Check sheet for the modelled part. Datum: model origin and axes. Units: mm. A direction names the side the tool comes from. Give positions to 0.01 mm unless a question says otherwise; leave off trailing zeros. Loops run counter-clockwise (first coordinate to the right, second up) from the corner with the lowest first, then second, coordinate; pieces in that order, holes last. Notation, with made-up numbers: (0.5, 2.25) - (4.5, 2.25) arc R23 ccw to (4.5, 17.25) - close; hole circle Ø4 at (-38, 84.25). An arc over 180 degrees is marked (long way). Use CSV: the item, a comma, the result in double quotes.
from build123d import *

# Parameters (mm, degrees)
SKETCH_R  = 1.7
PAD_DEPTH = 3


with BuildPart() as part:
    # Sketch → Pad (new body)
    with BuildSketch(Plane.XY):
        with BuildLine():
            ThreePointArc((-11.338775, -5.261385), (-11.137582, -5.674881), (-10.921315, -6.080698))
            Line((-10.921315, -6.080698), (-12.869031, -8.11383))
            ThreePointArc((-12.869031, -8.11383), (-12.957339, -9.414058), (-11.69346, -9.731864))
            Line((-11.69346, -9.731864), (-9.157959, -8.507749))
            ThreePointArc((-9.157959, -8.507749), (-8.838835, -8.838835), (-8.507749, -9.157959))
            Line((-8.507749, -9.157959), (-9.731864, -11.69346))
            ThreePointArc((-9.731864, -11.69346), (-9.414058, -12.957339), (-8.11383, -12.869031))
            Line((-8.11383, -12.869031), (-6.080698, -10.921315))
            ThreePointArc((-6.080698, -10.921315), (-5.674881, -11.137582), (-5.261385, -11.338775))
            Line((-5.261385, -11.338775), (-5.642075, -14.128453))
            ThreePointArc((-5.642075, -14.128453), (-4.949263, -15.232265), (-3.739962, -14.746487))
            Line((-3.739962, -14.746487), (-2.408215, -12.265826))
            ThreePointArc((-2.408215, -12.265826), (-1.955431, -12.346104), (-1.5, -12.409674))
            Line((-1.5, -12.409674), (-1, -15.180455))
            ThreePointArc((-1, -15.180455), (0, -16.016151), (1, -15.180455))
            Line((1, -15.180455), (1.5, -12.409674))
            ThreePointArc((1.5, -12.409674), (7.008593, -10.350344), (10.965856, -6))
            Line((30.259157, -5), (10.965856, -6))
            ThreePointArc((30.259157, -5), (35.006712, 0), (30.259157, 5))
            Line((10.965856, 6), (30.259157, 5))
            ThreePointArc((10.965856, 6), (-0.413709, 12.493152), (-11.338775, 5.261385))
            Line((-11.338775, 5.261385), (-14.128453, 5.642075))
            ThreePointArc((-14.128453, 5.642075), (-15.232265, 4.949263), (-14.746487, 3.739962))
            Line((-14.746487, 3.739962), (-12.265826, 2.408215))
            ThreePointArc((-12.265826, 2.408215), (-12.346104, 1.955431), (-12.409674, 1.5))
            Line((-12.409674, 1.5), (-15.180455, 1))
            ThreePointArc((-15.180455, 1), (-16.016151, 0), (-15.180455, -1))
            Line((-15.180455, -1), (-12.409674, -1.5))
            ThreePointArc((-12.409674, -1.5), (-12.346104, -1.955431), (-12.265826, -2.408215))
            Line((-12.265826, -2.408215), (-14.746487, -3.739962))
            ThreePointArc((-14.746487, -3.739962), (-15.232265, -4.949263), (-14.128453, -5.642075))
            Line((-14.128453, -5.642075), (-11.338775, -5.261385))
        make_face()
        Circle(SKETCH_R, mode=Mode.SUBTRACT)
        with Locations((7, 0)):
            Circle(SKETCH_R, mode=Mode.SUBTRACT)
        with Locations((-7, 0)):
            Circle(SKETCH_R, mode=Mode.SUBTRACT)
        with Locations((30, 0)):
            Circle(SKETCH_R, mode=Mode.SUBTRACT)
    extrude(amount=PAD_DEPTH)


solid = part.part
1. Release check for a two-part mould opening along Y. For faces 4 (the face through (-8.35, -1.03, 1.48)), 5 (the face through (-0.2, 12.5, 1.5)), 6 (the face through (-1.962, -12.345, 1.479)) record: released by +Y, released by -Y, zero draft, split by the parting line, or undercut.
Completed:
face 4,"undercut"
face 5,"released by +Y"
face 6,"released by -Y"
2. Sectioned sample at C-C, the plane z = 0.6. State how many separate pieces and enclosed holes the cut face has, and give its area (3 significant figures).
Completed:
separate pieces,"1"
enclosed holes,"4"
area,"747 mm²"
3. Sectioned sample at A-A, the plane x = 0. Record the boundary of the cut face in (y, z).
Completed:
outline,"(-16.02, 0) - (-1.7, 0) - (-1.7, 3) - (-16.02, 3) - close; (1.7, 0) - (12.5, 0) - (12.5, 3) - (1.7, 3) - close"
4. Sectioned sample at D-D, the plane x = -7.5. Record the boundary of the cut face in (y, z).
Completed:
outline,"(-12.28, 0) - (-1.62, 0) - (-1.62, 3) - (-12.28, 3) - close; (1.62, 0) - (10, 0) - (10, 3) - (1.62, 3) - close"
5. Set-up check for faces 1 (the face through (-12.347, -1.949, 1.479)), 2 (the face through (-12.753, -5.454, 1.479)), 3 (the face through (-3.08, -13.52, 1.48)): record each of +Z, -Z, +X, -X, +Y, -Y from which the full face is reachable in a straight line by a thin tool's end or side.
Completed:
face 1,"+Z, -Z, -X"
face 2,"+Z, -Z"
face 3,"+Z, -Z, -Y"
6. Scan lines: line 1 along Y through (x, z) = (0, 1.4); line 2 along Y through (x, z) = (7.5, 1.65); line 3 along X through (y, z) = (-13.5, 1.2). Record each from-to range of solid material in increasing order.
Completed:
line 1,"y = -16.02 to -1.7, 1.7 to 12.5"
line 2,"y = -10 to -1.62, 1.62 to 10"
line 3,"x = -5.56 to -3.07, -1.3 to 1.3"
7. Sectioned sample at B-B, the plane y = 0. Record the boundary of the cut face in (x, z), and give its area (3 significant figures).
Completed:
outline,"(-16.02, 0) - (-8.7, 0) - (-8.7, 3) - (-16.02, 3) - close; (-5.3, 0) - (-1.7, 0) - (-1.7, 3) - (-5.3, 3) - close; (1.7, 0) - (5.3, 0) - (5.3, 3) - (1.7, 3) - close; (8.7, 0) - (28.3, 0) - (28.3, 3) - (8.7, 3) - close; (31.7, 0) - (35.01, 0) - (35.01, 3) - (31.7, 3) - close"
area,"112 mm²"
